```python
from build123d import *

# Parameters (mm, degrees)
BOSS_EXTRUDE4_DEPTH = 254


with BuildPart() as part:
    # Sketch1 → Boss-Extrude4 (new body)
    with BuildSketch(Plane(origin=(0, 0, 0), x_dir=(0, 0, -1), z_dir=(1, 0, 0))):
        with BuildLine():
            Line((-76.879940582, 0), (-89.563831565, 0))
            Line((-89.563831565, 0), (-89.563831565, 3.175))
            Line((-89.563831565, 3.175), (-78.039725897, 3.175))
            ThreePointArc((-78.039725897, 3.175), (-63.553584925, 8.017140461), (-49.363273916, 2.366505276))
            ThreePointArc((-49.363273916, 2.366505276), (-38.779940582, -1.675968343), (-28.196607249, 2.366505276))
            ThreePointArc((-28.196607249, 2.366505276), (-13.379940582, 8.025968343), (1.436726084, 2.366505276))
            ThreePointArc((1.436726084, 2.366505276), (12.020059418, -1.675968343), (22.603392751, 2.366505276))
            ThreePointArc((22.603392751, 2.366505276), (37.905111105, 8.020674683), (52.945511479, 1.704142972))
            ThreePointArc((52.945511479, 1.704142972), (75.245720478, -15.063067291), (96.359970712, 3.175))
            Line((96.359970712, 3.175), (111.566304511, 3.175))
            Line((111.566304511, 3.175), (111.566304511, 0))
            Line((111.566304511, 0), (98.866304511, 0))
            ThreePointArc((98.866304511, 0), (74.493181964, -18.250811422), (50.120059418, 0))
            ThreePointArc((50.120059418, 0), (37.420059418, 4.850968343), (24.720059418, 0))
            ThreePointArc((24.720059418, 0), (12.020059418, -4.850968343), (-0.679940582, 0))
            ThreePointArc((-0.679940582, 0), (-13.379940582, 4.850968343), (-26.079940582, 0))
            ThreePointArc((-26.079940582, 0), (-38.779940582, -4.850968343), (-51.479940582, 0))
            ThreePointArc((-51.479940582, 0), (-64.179940582, 4.850968343), (-76.879940582, 0))
        make_face()
    extrude(amount=BOSS_EXTRUDE4_DEPTH)


solid = part.part
```
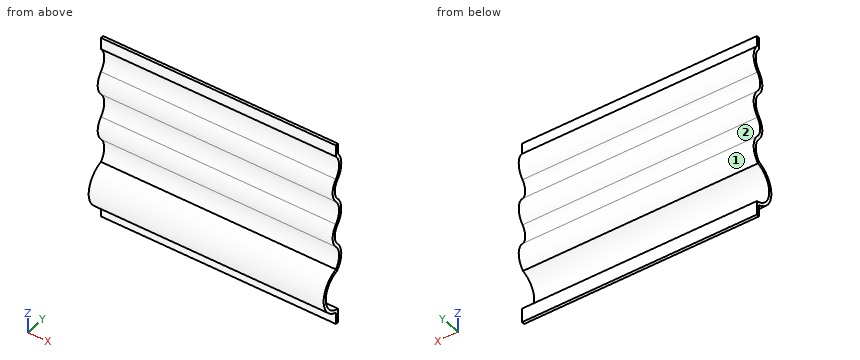
Input: part model. Units: mm. Frame: model coordinates. Face numbers are marked on the shaded views. Give positions to 0.01 mm unless a question says otherwise; leave off trailing zeros. Write each loop counter-clockwise with the first axis right and the second up, starting at its lowest first coordinate (ties: lowest second). Pieces come first, ordered by that corner, then holes. Notation, with made-up numbers: (85.5, 36.25) - (109.5, 36.25) arc R24 ccw to (109.5, 55.25) - close; hole circle Ø2 at (14.5, -17). An arc over 180 degrees is marked (long way). Write item = value, one per line. Start each with the question number.
1. Ray query, L1, parallel to Z at x = 143, y = 5; L2, parallel to Z at x = 25, y = 3.5; L3, parallel to Z at x = 188, y = -10.5. Return the intervals inside material, ascending.
2. Section query C-C, the plane z = -59. Output: boundary loops of the cut face in (x, y).
3. Section query B-B, the plane y = -9. Output: boundary loops of the cut face in (x, z), then the cut area to 3 significant figures.
4. Mould query, pull axis Z, two halves, no side actions, for the marked faces 1 and 2. Classes: released by +Z, released by -Z, zero draft, split by the parting line, or undercut.
5. Section query D-D, the plane z = 34. Output: boundary loops of the cut face in (x, y), then the cut area to 3 significant figures.
6. First-contact query: pin 1 Ø9 at (x, z) = (177, 85.5) entering from +Y (3 decimals); pin 2 Ø10 at (x, y) = (33.5, -12.5) entering from -Z; pin 3 Ø4 at (x, y) = (28.5, -12.5) entering from -Z. Flat tips, straight axial feed; report the tip coordinate or a pass-through.
Check sheet entries:
q1.L1 = -48.62 to -26.22, 2.18 to 24.58, 52.98 to 75.38
q1.L2 = -50.86 to -44.47, -30.37 to -23.98, -0.06 to 6.33, 20.43 to 26.82, 50.74 to 57.13, 71.23 to 77.62
q1.L3 = -92.76 to -88, -60.99 to -56.23
q2.outline = (0, -12.98) - (254, -12.98) - (254, -8.79) - (0, -8.79) - close
q3.outline = (0, -94.1) - (254, -94.1) - (254, -89.76) - (0, -89.76) - close; (0, -59.22) - (254, -59.22) - (254, -54.89) - (0, -54.89) - close
q3.area = 2,200 mm2
q4.face_1 = undercut
q4.face_2 = undercut
q5.outline = (0, -4.24) - (254, -4.24) - (254, -0.94) - (0, -0.94) - close
q5.area = 839 mm2
q6.pin_1 = 3.175
q6.pin_2 = -95.24
q6.pin_3 = -92.76
